```python
from build123d import *

# Parameters (mm, degrees)
F0_R          = 15
F1_DEPTH      = 550
F2_R          = 35
F3_DEPTH      = 15
F3_DEPTH_BACK = 15
F4_R          = 15
F5_DEPTH      = 30.001


with BuildPart() as f1:
    # F0 (on Front) → F1 (new body)
    with BuildSketch(Plane.XZ):
        Circle(F0_R)
    extrude(amount=-F1_DEPTH)

    # F2 (on Right) → F3 (join, two sides)
    with BuildSketch(Plane.YZ) as f3_sk:
        with Locations((-31, 0)):
            Circle(F2_R)
    extrude(amount=F3_DEPTH)
    extrude(f3_sk.sketch, amount=-F3_DEPTH_BACK)

    # F4 (on face) → F5 (cut, through all)
    with BuildSketch(Plane.YZ.offset(15)):
        with Locations((-31, 0)):
            Circle(F4_R)
    extrude(amount=-F5_DEPTH, mode=Mode.SUBTRACT)


solid = f1.part
```
Verification items for the finished model (mm, model axes). Round coordinates to 2 decimals unless told otherwise and drop trailing zeros. Write each loop counter-clockwise with the first axis right and the second up, starting at its lowest first coordinate (ties: lowest second). Pieces come first, ordered by that corner, then holes.
1. Draft check along Z on faces 1 (the cylindrical face through (0.21, -45.985, 0.66)), 2 (the cylindrical face through (-14.985, 271.466, 0.66)), 3 (the flat face through (0, 550, 0)). Enter one of: +Z half, -Z half, draft (parallel to the pull), parting line (faces both ways), or undercut.
2. Section check D-D on y = 76. Enter the section's corners in (x, z), plus the area to 3 significant figures.
3. Section check C-C on z = 28. Enter the section's corners in (x, y).
4. Section check B-B on z = 5.5. Enter the section's corners in (x, y), plus the area to 3 significant figures.
5. Section check A-A on y = -31. Enter the section's corners in (x, z).
6. Gauge pin test, flat ends, axial feed: P1, Ø3, axis at y = 340.5, z = 2, coming from the -X side; P2, Ø1, axis at x = -2.5, y = 165, coming from the -Z side; P3, Ø1.5, axis at x = -2.5, z = -24.5, coming from the +Y side. Record the tip position at first contact, or that the pin passes through.
7. Scan lines: L1, parallel to Z at x = 6, y = -31; L2, parallel to Y at x = 10, z = 1; L3, parallel to Y at x = -12, z = 2. Record each from-to range of solid material in increasing order.
Answer:
1. face 1: undercut
1. face 2: parting line
1. face 3: draft
2. outline: circle Ø30 at (0, 0)
2. area: 707 mm2
3. outline: (-15, -52) - (15, -52) - (15, -10) - (-15, -10) - close
4. outline: (-15, -65.57) - (15, -65.57) - (15, -44.96) - (-15, -44.96) - close; (-15, -17.04) - (15, -17.04) - (15, 3.57) - (13.96, 3.57) - (13.96, 550) - (-13.96, 550) - (-13.96, 3.57) - (-15, 3.57) - close
4. area: 16,500 mm2
5. outline: (-15, -35) - (15, -35) - (15, -15) - (-15, -15) - close; (-15, 15) - (15, 15) - (15, 35) - (-15, 35) - close
6. P1: stops at x = -14.99
6. P2: stops at z = -14.87
6. P3: stops at y = -5.29
7. L1: z = -35 to -15, 15 to 35
7. L2: y = -65.99 to -45.97, -16.03 to 550
7. L3: y = -65.94 to -45.87, -16.13 to 550
